from build123d import *

# Parameters (mm, degrees)
ESQUISSE1_W             = 100
ESQUISSE1_H             = 90
BOSS_EXTRU_1_DEPTH      = 3
ENL_V_MAT_EXTRU_1_REACH = 90.04
ESQUISSE2_W             = 40
ESQUISSE2_H             = 3
ESQUISSE2_W_2           = 3
ESQUISSE2_H_2           = 30


with BuildPart() as part:
    # Esquisse1 → Boss.-Extru.1 (new body)
    with BuildSketch(Plane.XY):
        with Locations((-10.038524431, -19.32304038)):
            Rectangle(ESQUISSE1_W, ESQUISSE1_H)
    extrude(amount=BOSS_EXTRU_1_DEPTH)

    # Esquisse2 → Enlèv. mat.-Extru.1 (cut, up to next)
    with BuildSketch(Plane.XY.offset(3), mode=Mode.PRIVATE) as enl_v_mat_extru_1_sk1:
        with Locations((-10.038524431, 24.17695962)):
            Rectangle(ESQUISSE2_W, ESQUISSE2_H)
    enl_v_mat_extru_1_tool1 = extrude(enl_v_mat_extru_1_sk1.sketch, amount=-ENL_V_MAT_EXTRU_1_REACH, mode=Mode.PRIVATE) & part.part
    # Esquisse2 → Enlèv. mat.-Extru.1 (cut, up to next)
    with BuildSketch(Plane.XY.offset(3), mode=Mode.PRIVATE) as enl_v_mat_extru_1_sk2:
        with Locations((-58.538524431, 10.67695962)):
            Rectangle(ESQUISSE2_W_2, ESQUISSE2_H_2)
    enl_v_mat_extru_1_tool2 = extrude(enl_v_mat_extru_1_sk2.sketch, amount=-ENL_V_MAT_EXTRU_1_REACH, mode=Mode.PRIVATE) & part.part
    # Esquisse2 → Enlèv. mat.-Extru.1 (cut, up to next)
    with BuildSketch(Plane.XY.offset(3), mode=Mode.PRIVATE) as enl_v_mat_extru_1_sk3:
        with Locations((-58.538524431, -49.32304038)):
            Rectangle(ESQUISSE2_W_2, ESQUISSE2_H_2)
    enl_v_mat_extru_1_tool3 = extrude(enl_v_mat_extru_1_sk3.sketch, amount=-ENL_V_MAT_EXTRU_1_REACH, mode=Mode.PRIVATE) & part.part
    # Esquisse2 → Enlèv. mat.-Extru.1 (cut, up to next)
    with BuildSketch(Plane.XY.offset(3), mode=Mode.PRIVATE) as enl_v_mat_extru_1_sk4:
        with Locations((-10.038524431, -62.82304038)):
            Rectangle(ESQUISSE2_W, ESQUISSE2_H)
    enl_v_mat_extru_1_tool4 = extrude(enl_v_mat_extru_1_sk4.sketch, amount=-ENL_V_MAT_EXTRU_1_REACH, mode=Mode.PRIVATE) & part.part
    # Esquisse2 → Enlèv. mat.-Extru.1 (cut, up to next)
    with BuildSketch(Plane.XY.offset(3), mode=Mode.PRIVATE) as enl_v_mat_extru_1_sk5:
        with Locations((38.461475569, -49.32304038)):
            Rectangle(ESQUISSE2_W_2, ESQUISSE2_H_2)
    enl_v_mat_extru_1_tool5 = extrude(enl_v_mat_extru_1_sk5.sketch, amount=-ENL_V_MAT_EXTRU_1_REACH, mode=Mode.PRIVATE) & part.part
    # Esquisse2 → Enlèv. mat.-Extru.1 (cut, up to next)
    with BuildSketch(Plane.XY.offset(3), mode=Mode.PRIVATE) as enl_v_mat_extru_1_sk6:
        with Locations((38.461475569, 10.67695962)):
            Rectangle(ESQUISSE2_W_2, ESQUISSE2_H_2)
    enl_v_mat_extru_1_tool6 = extrude(enl_v_mat_extru_1_sk6.sketch, amount=-ENL_V_MAT_EXTRU_1_REACH, mode=Mode.PRIVATE) & part.part
    add(enl_v_mat_extru_1_tool1.solids().sort_by_distance((-10.038524, 24.17696, 3))[0], mode=Mode.SUBTRACT)
    add(enl_v_mat_extru_1_tool2.solids().sort_by_distance((-58.538524, 10.67696, 3))[0], mode=Mode.SUBTRACT)
    add(enl_v_mat_extru_1_tool3.solids().sort_by_distance((-58.538524, -49.32304, 3))[0], mode=Mode.SUBTRACT)
    add(enl_v_mat_extru_1_tool4.solids().sort_by_distance((-10.038524, -62.82304, 3))[0], mode=Mode.SUBTRACT)
    add(enl_v_mat_extru_1_tool5.solids().sort_by_distance((38.461476, -49.32304, 3))[0], mode=Mode.SUBTRACT)
    add(enl_v_mat_extru_1_tool6.solids().sort_by_distance((38.461476, 10.67696, 3))[0], mode=Mode.SUBTRACT)


solid = part.part
For this review, take the finished solid that the model builds, in its own axes (mm). A direction names the side the tool comes from. Round coordinates to 2 decimals unless told otherwise and drop trailing zeros. Loops run counter-clockwise (first coordinate to the right, second up) from the corner with the lowest first, then second, coordinate; pieces in that order, holes last. Notation, with made-up numbers: (58.5, 40.25) - (100.5, 40.25) arc R12 cw to (100.5, 44.25) - close; hole circle Ø10 at (71, 22.25). An arc over 180 degrees is marked (long way). Use one line per item in the form item = value.
Item 1: Consider section C-C on y = -52.5. Write out the cut boundary in (x, z), then the cut area to 3 significant figures.
Answers:
outline = (-57.04, 0) - (36.96, 0) - (36.96, 3) - (-57.04, 3) - close
area = 282 mm^2
Item 2: Mouldability with a two-part tool opening along X and no side actions: class faces 1 (the flat face through (-30.039, -63, 2)), 2 (the flat face through (-30.039, 24, 2)), 3 (the flat face through (39.961, -20, 1)), 4 (the flat face through (-44, -64.323, 1)) as +X half, -X half, draft (parallel to the pull), parting line (faces both ways), or undercut.
Answers:
face_1 = undercut
face_2 = undercut
face_3 = +X half
face_4 = draft
Item 3: Consider section B-B on x = -28. Write out the cut boundary in (y, z).
Answers:
outline = (-61.32, 0) - (22.68, 0) - (22.68, 3) - (-61.32, 3) - close
Item 4: For line 1 (Y direction, x = -11, z = 1.6); line 2 (X direction, y = -47, z = 2.55), list the stretches that pass through material, from the lowest coordinate up.
Answers:
line_1 = -61.32 to 22.68
line_2 = -57.04 to 36.96
Item 5: Clearance check with flat-ended pins moving along their axes: P1, Ø0.9, axis at y = 9.5, z = 1, coming from the -X side; P2, Ø1.5, axis at x = -15, z = 1.5, coming from the -Y side; P3, Ø1.5, axis at y = 12.5, z = 2, coming from the +X side. State where each tip first meets the part, or that it passes through.
Answers:
P1 = -57.04
P2 = -61.32
P3 = 36.96
Item 6: Tool access review of faces 5 (the flat face through (36.961, -50, 2)), 6 (the flat face through (-57.039, -50, 2)), 7 (the flat face through (-10, 22.677, 2)): name each direction out of +Z, -Z, +X, -X, +Y, -Y from which nothing blocks a thin tool from reaching the whole face with its end or side.
Answers:
face_5 = +Z, -Z, +X, -Y
face_6 = +Z, -Z, -X, -Y
face_7 = +Z, -Z, +Y
Item 7: Consider section A-A on z = 1.2. Write out the cut boundary in (x, y).
Answers:
outline = (-60.04, -34.32) - (-57.04, -34.32) - (-57.04, -64.32) - (-30.04, -64.32) - (-30.04, -61.32) - (9.96, -61.32) - (9.96, -64.32) - (36.96, -64.32) - (36.96, -34.32) - (39.96, -34.32) - (39.96, -4.32) - (36.96, -4.32) - (36.96, 25.68) - (9.96, 25.68) - (9.96, 22.68) - (-30.04, 22.68) - (-30.04, 25.68) - (-57.04, 25.68) - (-57.04, -4.32) - (-60.04, -4.32) - close
